The model under review builds one solid part; all positions refer to its coordinate system, in mm. Face numbers are marked on the shaded views. A direction names the side the tool comes from. Round coordinates to 2 decimals unless told otherwise and drop trailing zeros. Write each loop counter-clockwise with the first axis right and the second up, starting at its lowest first coordinate (ties: lowest second). Pieces come first, ordered by that corner, then holes. Notation, with made-up numbers: (-29, 79) -> (-19, 79) arc R22 cw to (-19, 101) -> close; hole circle Ø6 at (35.25, 69.5). An arc over 180 degrees is marked (long way). Return JSON: item names as keys, results as strings. Group by question number.
1. Take a section at D-D, the plane x = -7. Write out the cut boundary in (y, z).
2. Take a section at B-B, the plane x = 3. Write out the cut boundary in (y, z).
3. Take a section at C-C, the plane z = -90. Give the number of separate pieces and of enclosed holes in the cut face, then the cut area to 3 significant figures.
4. Clearance check with flat-ended pins moving along their axes: P1, Ø16.5, axis at x = -21, z = -43.5, coming from the +Y side; P2, Ø1.5, axis at y = 20, z = -104, coming from the +X side; P3, Ø16, axis at x = 33.5, z = -84, coming from the +Y side. State where each tip first meets the part, or that it passes through.
5. For line 1 along X through (y, z) = (-17, -10); line 2 along Y through (x, z) = (20.5, -34); line 3 along Y through (x, z) = (-20.5, -47), list the stretches that pass through material, from the lowest coordinate up. Write a range as from..to.
6. Take a section at A-A, the plane x = -19. Write out the cut boundary in (y, z), then the cut area to 3 significant figures.
7. Tool access review of the marked faces 5, 6, 7 and 8: name each direction out of +Z, -Z, +X, -X, +Y, -Y from which nothing blocks a thin tool from reaching the whole face with its end or side.
8. Mouldability with a two-part tool opening along Z and no side actions: class the marked faces 1, 2, 3 and 4 as pulls with the +Z half, pulls with the -Z half, needs draft (parallel to the pull), parting line crosses it, or undercut.
from build123d import *

# Parameters (mm, degrees)
SKETCH_1_W          = 6
SKETCH_1_H          = 6
EXTRUDE_1_DEPTH     = 40
EXTRUDE_2_DEPTH     = 10
EXTRUDE_4_DEPTH     = 25
EXTRUDE_5_DEPTH     = 25
FILLET_4_R          = 10
FILLET_5_R          = 10
FILLET_6_R          = 10
FILLET_7_R          = 10
CUT_EXTRUDE_1_DEPTH = 30
FILLET_11_R         = 10
SKETCH_5_R          = 2.099999999999999
SKETCH_5_R_2        = 2.0999999999999983
SKETCH_5_R_3        = 2.1
SKETCH_5_R_4        = 2.0999999999999965
CUT_EXTRUDE_2_DEPTH = 255.61889299989065
CUT_EXTRUDE_3_DEPTH = 255.61889299989065
CUT_EXTRUDE_4_DEPTH = 240.03655739851368
EXTRUDE_6_DEPTH     = 16
SKETCH_5_2_R        = 2.099999999999999
SKETCH_5_2_R_2      = 2.0999999999999983
SKETCH_5_2_R_3      = 2.1
SKETCH_5_2_R_4      = 2.0999999999999965
CUT_EXTRUDE_5_DEPTH = 179.3042624280185


with BuildPart() as part:
    # Sketch 1 → Extrude 1 (new body)
    with BuildSketch(Plane(origin=(0, 0, 0), x_dir=(0, 0, -1), z_dir=(1, 0, 0))):
        Polygon((113.39745962155384, 1.22e-15), (0, 0), (0, -6), (6, -6), (135.7897644669674, -5.999999999999998), (23.38853128737442, 58.894882233482974), (18.192378864667774, 61.89488223348294), (15.192378864667806, 56.69872981077631), align=None)
        Polygon((40.19237886466755, 99.99999999999838), (37.19237886466758, 94.80384757729173), (42.38853128737424, 91.80384757729176), (224.71796769724395, -13.464101615137775), (224.71796769724395, -6.5358983848622865), align=None)
        Polygon((6.000000000000005, -44.00000000000001), (5.33e-15, -44.00000000000001), (0, -50), (224.71796769724395, -50), (224.71796769724395, -44.00000000000001), align=None)
        with Locations((227.71796769724392, -47.00000000000001)):
            Rectangle(SKETCH_1_W, SKETCH_1_H)
        Polygon((224.71796769724395, -13.464101615137768), (224.71796769724395, -44.00000000000001), (230.71796769724395, -44.00000000000001), (230.71796769724395, -16.92820323027548), align=None)
        Polygon((224.71796769724395, -6.5358983848622865), (224.71796769724395, -13.464101615137768), (230.71796769724395, -16.92820323027548), (230.71796769724395, -10.000000000000002), align=None)
    extrude(amount=EXTRUDE_1_DEPTH)

    # Sketch 1_6 → Extrude 2 (add)
    with BuildSketch(Plane(origin=(0, 0, 0), x_dir=(0, 0, -1), z_dir=(1, 0, 0))):
        Polygon((6, -6), (0, -6), (0, -44.00000000000001), (6.000000000000005, -44.00000000000001), (224.71796769724395, -44.00000000000001), (224.71796769724395, -13.464101615137768), (42.388531287374235, 91.80384757729178), (37.192378864667575, 94.80384757729173), (18.192378864667766, 61.89488223348294), (23.38853128737442, 58.89488223348298), (135.7897644669674, -5.999999999999998), align=None)
    extrude(amount=EXTRUDE_2_DEPTH)

    # Sketch 1_9 → Extrude 4 (add)
    with BuildSketch(Plane(origin=(0, 0, 0), x_dir=(0, 0, -1), z_dir=(1, 0, 0))):
        Polygon((6.000000000000005, -44.00000000000001), (5.33e-15, -44.00000000000001), (0, -50), (224.71796769724395, -50), (224.71796769724395, -44.00000000000001), align=None)
    extrude(amount=-EXTRUDE_4_DEPTH)

    # Sketch 2 → Extrude 5 (add)
    with BuildSketch(Plane.ZY):
        Polygon((0, 0), (-213.3974596215552, -2.429e-14), (-223.78976446696848, -6.0000000000000275), (0, -6), align=None)
    extrude(amount=EXTRUDE_5_DEPTH)

    # Fillet 4
    fillet_4_edges = [part.edges().sort_by_distance(p)[0] for p in [
        (20, 1.22e-15, -113.39745962155384),
        (0, -1.86e-14, -163.39745962155453),
    ]]
    fillet(fillet_4_edges, radius=FILLET_4_R)

    # Fillet 5
    fillet_5_edges = [part.edges().sort_by_distance(p)[0] for p in [
        (0, -44.00000000000001, -112.35898384862197),
        (0, -6.000000000000014, -111.89488223348424),
    ]]
    fillet(fillet_5_edges, radius=FILLET_5_R)

    # Fillet 6
    fillet_6_edges = [part.edges().sort_by_distance(p)[0] for p in [
        (25, -13.464101615137771, -224.71796769724395),
        (25, -44.00000000000001, -224.71796769724395),
    ]]
    fillet(fillet_6_edges, radius=FILLET_6_R)

    # Fillet 7
    fillet_7_edges = [part.edges().sort_by_distance(p)[0] for p in [
        (18.999999999999993, -10.000000000000007, -230.71796769724395),
    ]]
    fillet(fillet_7_edges, radius=FILLET_7_R)

    # Sketch 3 → Cut-Extrude 1 (cut)
    with BuildSketch(Plane(origin=(40, 0, 0), x_dir=(0, 0, -1), z_dir=(1, 0, 0))):
        with BuildLine():
            Line((101.0769515458646, -5.999999999999998), (135.7897644669674, -5.999999999999998))
            Line((135.7897644669674, -5.999999999999998), (105.72758664047566, 11.356406460551396))
            ThreePointArc((105.72758664047566, 11.356406460551396), (110.06128863892687, 0.8939243206071232), (101.0769515458646, -5.999999999999998))
        make_face()
    extrude(amount=-CUT_EXTRUDE_1_DEPTH, mode=Mode.SUBTRACT)

    # Fillet 11
    fillet_11_edges = [part.edges().sort_by_distance(p)[0] for p in [
        (10, -44.00000000000001, -107.35898384862197),
        (10, -26.618802153516928, -224.71796769724395),
        (10, 42.11324865405107, -128.45517328095568),
        (10, -14.23760430703381, -223.3782217350883),
        (10, -41.07106781186548, -221.78903550910942),
        (10, 36.62564434701707, -61.95998275257166),
        (10, 0.8939243206071223, -110.06128863892687),
        (10, -5.999999999999999, -50.5384757729323),
    ]]
    fillet(fillet_11_edges, radius=FILLET_11_R)

    # Sketch 5 → Cut-Extrude 2 (cut, through all)
    with BuildSketch(Plane(origin=(0, 0, 0), x_dir=(1, 0, 0), z_dir=(0, 1, 1e-17))):
        with Locations(Location((-15.000000000000002, 10, 0), (0, 0, 270))):
            Circle(SKETCH_5_R)
        with Locations(Location((-15.000000000000139, 50, 0), (0, 0, 270))):
            Circle(SKETCH_5_R_2)
        with Locations(Location((-15.000000000000275, 90, 0), (0, 0, 270))):
            Circle(SKETCH_5_R_3)
        with Locations(Location((-15.000000000000412, 130, 0), (0, 0, 270))):
            Circle(SKETCH_5_R_4)
    extrude(amount=-CUT_EXTRUDE_2_DEPTH, mode=Mode.SUBTRACT)

    # Sketch 6 → Cut-Extrude 3 (cut, through all)
    with BuildSketch(Plane(origin=(0, 0, 0), x_dir=(1, 0, 0), z_dir=(0, 1, 1e-17))):
        Polygon((-25, 231.5180230769059), (40, 231.5180230769059), (40.00000000000001, 142.1), (-24.99999999999999, 142.1), align=None)
    extrude(amount=-CUT_EXTRUDE_3_DEPTH, mode=Mode.SUBTRACT)

    # Sketch 6_2 → Cut-Extrude 4 (cut, through all)
    with BuildSketch(Plane(origin=(0, 0, 0), x_dir=(1, 0, 0), z_dir=(0, 1, 1e-17))):
        Polygon((-25, 231.5180230769059), (40, 231.5180230769059), (40.00000000000001, 142.1), (-24.99999999999999, 142.1), align=None)
    extrude(amount=CUT_EXTRUDE_4_DEPTH, mode=Mode.SUBTRACT)

    # Sketch 8 → Extrude 6 (add)
    with BuildSketch(Plane.XZ.offset(6)):
        Polygon((-25, -7.4e-16), (-24.99999999999999, -142.1), (0, -142.1), (0, 0), align=None)
    extrude(amount=EXTRUDE_6_DEPTH)

    # Sketch 5_2 → Cut-Extrude 5 (cut, through all)
    with BuildSketch(Plane(origin=(0, 0, 0), x_dir=(1, 0, 0), z_dir=(0, 1, 1e-17))):
        with Locations(Location((-15.000000000000002, 10, 0), (0, 0, 270))):
            Circle(SKETCH_5_2_R)
        with Locations(Location((-15.000000000000139, 50, 0), (0, 0, 270))):
            Circle(SKETCH_5_2_R_2)
        with Locations(Location((-15.000000000000275, 90, 0), (0, 0, 270))):
            Circle(SKETCH_5_2_R_3)
        with Locations(Location((-15.000000000000412, 130, 0), (0, 0, 270))):
            Circle(SKETCH_5_2_R_4)
    extrude(amount=-CUT_EXTRUDE_5_DEPTH, mode=Mode.SUBTRACT)


solid = part.part
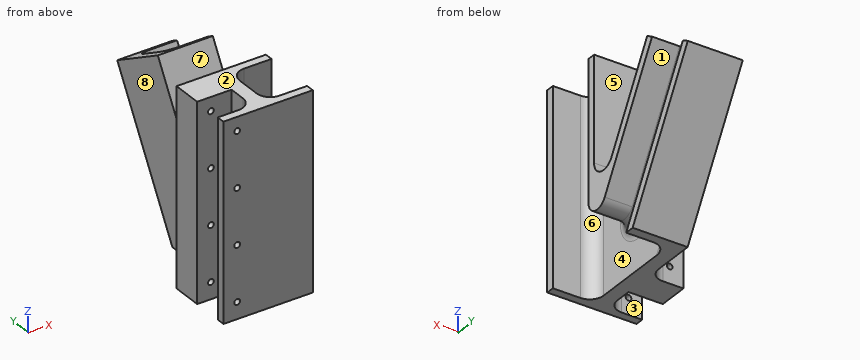
Output:
{
 "1": {"outline": "(-50, -142.1) -> (-43.54, -142.1) -> (-43.54, 0) -> (-50, 0) -> close; (-22, -142.1) -> (0.46, -142.1) -> (0.46, -79.08) arc R10 cw to (0, -76.08) -> (0, 0) -> (-22, 0) -> close"},
 "2": {"outline": "(-50, -142.1) -> (41.16, -142.1) -> (100, -40.19) -> (56.7, -15.19) -> (18.66, -81.08) arc R10 cw to (0, -76.08) -> (0, 0) -> (-50, 0) -> close"},
 "3": {"separate pieces": "3", "enclosed holes": "0", "area": "3,110 mm^2"},
 "4": {"P1": "stops at y = 0", "P2": "stops at x = 10.89", "P3": "stops at y = 79.33"},
 "5": {"line 1": "x = -25..-17.1, -12.9..10", "line 2": "y = -50..-44, -6..0, 45.84..52.77", "line 3": "y = -50..-44, -22..0"},
 "6": {"outline": "(-50, -142.1) -> (-44, -142.1) -> (-44, 0) -> (-50, 0) -> close; (-22, -142.1) -> (0, -142.1) -> (0, 0) -> (-22, 0) -> close", "area": "3,980 mm^2"},
 "7": {"face 5": "+Z, -X", "face 6": "+Z, -Z, +X", "face 7": "+Z, +X, -X", "face 8": "+Z, -Z, -X, +Y"},
 "8": {"face 1": "undercut", "face 2": "pulls with the +Z half", "face 3": "needs draft", "face 4": "undercut"}
}
